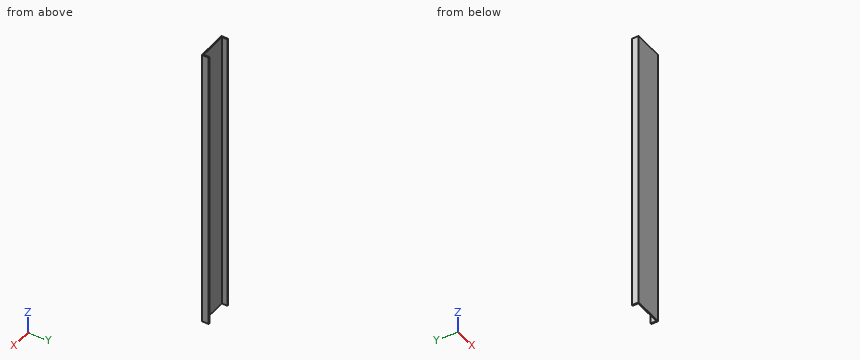
Autodesk Inventor part; units mm, degrees
ref_plane "YZ Plane" through (0, 0, 0) normal (1, 0, 0) x (0, 1, 0)
ref_plane "XZ Plane" through (0, 0, 0) normal (0, 1, 0) x (-1, 0, 0)
ref_plane "XY Plane" through (0, 0, 0) normal (0, 0, 1) x (1, 0, 0)
sketch "Sketch1" plane through (0, 0, 0) normal (0, 0, 1) x (1, 0, 0)
  line L0 (0, 0) -> (0, 19.05)
  line L1 (0, 19.05) -> (3.175, 19.05)
  line L2 (3.175, 19.05) -> (3.175, 3.175)
  line L3 (3.175, 3.175) -> (82.55, 3.175)
  line L4 (0, 0) -> (85.725, 0)
  line L5 (0, 0) -> (85.725, 0) construction
  line L6 (85.725, 0) -> (85.725, 19.05)
  line L7 (82.55, 3.175) -> (82.55, 19.05)
  line L8 (82.55, 19.05) -> (85.725, 19.05)
  dimension "d7" = 19.05
  dimension "d8" = 3.175
  dimension "d9" = 15.875
  dimension "d10" = 79.375
  dimension "d11" = 90
  dimension "d12" = 85.725
  dimension "d13" = 0
  dimension "d14" = 19.05
extrude "Extrusion1" add sketch "Sketch1" along normal blind 812.8
properties part number "FrameSide"
The model under review builds one solid part; all positions refer to its coordinate system, in mm. Give positions to 0.01 mm unless a question says otherwise; leave off trailing zeros. Loops run counter-clockwise (first coordinate to the right, second up) from the corner with the lowest first, then second, coordinate; pieces in that order, holes last. Notation, with made-up numbers: (41.5, -13) -> (98.5, -13) arc R29 cw to (98.5, 11) -> close; hole circle Ø7 at (50, -38.5). An arc over 180 degrees is marked (long way). Use CSV: the item, a comma, the result in double quotes.
1. Consider section C-C, the plane x = 23.5. Write out the cut boundary in (y, z) (3 decimals), then the cut area to 3 significant figures.
Result:
outline,"(0, 0) -> (3.175, 0) -> (3.175, 812.8) -> (0, 812.8) -> close"
area,"2,580 mm²"
2. Consider section B-B, the plane z = 160.5. Write out the cut boundary in (x, y) (3 decimals).
Result:
outline,"(0, 0) -> (85.725, 0) -> (85.725, 19.05) -> (82.55, 19.05) -> (82.55, 3.175) -> (3.175, 3.175) -> (3.175, 19.05) -> (0, 19.05) -> close"
3. For P1, Ø3, axis at x = 56, z = 558, coming from the +Y side (3 decimals), flat-tipped, find the tip position at first contact; note if it passes through.
Result:
P1,"stops at y = 3.175"
4. To check wall thickness, follow probe 1 along X at (y, z) = (9.5, 363) (3 decimals); probe 2 along Y at (x, z) = (47.5, 706) (3 decimals). State the ranges of each line that lie inside material, in increasing order. Write a range as from..to.
Result:
probe 1,"x = 0..3.175, 82.55..85.725"
probe 2,"y = 0..3.175"
5. Consider section A-A, the plane y = 9.5. Write out the cut boundary in (x, z) (3 decimals).
Result:
outline,"(0, 0) -> (3.175, 0) -> (3.175, 812.8) -> (0, 812.8) -> close; (82.55, 0) -> (85.725, 0) -> (85.725, 812.8) -> (82.55, 812.8) -> close"
